from build123d import *
from build123d import SkipClean  # not in build123d's __all__

# Parameters (mm, degrees)
F1_DEPTH = 30.1625
F0_R     = 26.9169820067
F2_DEPTH = 38.1
F6_D     = 4.7625
F6_DEPTH = 114.301
F7_D     = 17.4625
F7_DEPTH = 19.0282397391


with BuildPart() as f1:
    # F0 (on Front) → F1 (new body, symmetric)
    with BuildSketch(Plane.XZ):
        with BuildLine():
            ThreePointArc((41.2750103626, 4.8735072878), (43.5200676937, 3.9435676542), (44.4499999995, 1.6985072878))
            Line((44.4499999995, 1.6985072878), (44.4499999995, 0))
            Line((44.4499999995, 0), (88.8999999995, 0))
            Line((88.8999999995, 0), (88.8999999995, 13.5279764081))
            ThreePointArc((88.8999999995, 13.5279764081), (88.0492603051, 16.7029781548), (85.7249965061, 19.0272397391))
            Line((85.7249965061, 19.0272397391), (47.6269838993, 19.0272397391))
            ThreePointArc((47.6269838993, 19.0272397391), (40.8967892902, 21.812053872), (38.1019943796, 28.5381099704))
            Line((38.1019943796, 28.5381099704), (38.0289897107, 77.7511383134))
            ThreePointArc((38.0289897107, 77.7511383134), (-2e-10, 39.7221486024), (-38.0289897112, 77.7511383134))
            Line((-38.0289897112, 77.7511383134), (-38.0289897112, 31.7225298162))
            ThreePointArc((-38.0289897112, 31.7225298162), (-40.8187976204, 24.9873377254), (-47.5539897112, 22.1975298162))
            Line((-47.5539897112, 22.1975298162), (-82.55, 22.1975298162))
            ThreePointArc((-82.55, 22.1975298162), (-87.0401280605, 20.3376578767), (-88.9, 15.8475298162))
            Line((-88.9, 15.8475298162), (-88.9, 0))
            Line((-88.9, 0), (-44.45, 0))
            Line((-44.45, 0), (-44.45, 1.6987767268))
            ThreePointArc((-44.45, 1.6987767268), (-43.5200603664, 3.943844421), (-41.274989637, 4.8737767268))
            Line((-41.274989637, 4.8737767268), (41.2750103626, 4.8735072878))
        make_face()
    extrude(amount=F1_DEPTH, both=True)

    # F0 (on Front) → F2 (join, symmetric)
    with BuildSketch(Plane.XZ):
        with BuildLine():
            ThreePointArc((-38.0289897112, 77.7511383134), (-2e-10, 39.7221486024), (38.0289897107, 77.7511383134))
            ThreePointArc((38.0289897107, 77.7511383134), (-2e-10, 115.7801280244), (-38.0289897112, 77.7511383134))
        make_face()
        with Locations((-2e-10, 77.7511383134)):
            Circle(F0_R, mode=Mode.SUBTRACT)
    with SkipClean():  # cleaning this boolean's faces spoils the solid; the shape is the same uncleaned
        extrude(amount=F2_DEPTH, both=True)

    # F6 (through all, one way)
    with BuildSketch(Plane.XY.offset(114.3)):
        with Locations((0, 0)):
            Circle(F6_D / 2)
    extrude(amount=-F6_DEPTH, mode=Mode.SUBTRACT)

    # F7 (through all, one way)
    with BuildSketch(Plane.XY.offset(19.0272397391)):
        with Locations((-66.6769838993, 0), (66.6769838993, 0)):
            Circle(F7_D / 2)
    extrude(amount=-F7_DEPTH, mode=Mode.SUBTRACT)


solid = f1.part
The listing builds one solid part. Answer for the finished solid, in the listing's coordinates (mm). A direction names the side the tool comes from. Give positions to 0.01 mm unless a question says otherwise; leave off trailing zeros. Loops run counter-clockwise (first coordinate to the right, second up) from the corner with the lowest first, then second, coordinate; pieces in that order, holes last. Notation, with made-up numbers: (74, 25.5) - (98, 25.5) arc R15 ccw to (98, 30.5) - close; hole circle Ø5 at (57, -27). An arc over 180 degrees is marked (long way). Write each question's results on one line, items separated by ' | '.
1. Find section A-A, the plane x = 0. Write down the section's boundary in (y, z).
Resolved:
outline: (-38.1, 39.72) - (-30.16, 39.72) - (-30.16, 4.87) - (-2.38, 4.87) - (-2.38, 50.83) - (-38.1, 50.83) - close; (-38.1, 104.67) - (-2.38, 104.67) - (-2.38, 114.3) - (2.38, 114.3) - (2.38, 104.67) - (38.1, 104.67) - (38.1, 115.78) - (-38.1, 115.78) - close; (2.38, 4.87) - (30.16, 4.87) - (30.16, 39.72) - (38.1, 39.72) - (38.1, 50.83) - (2.38, 50.83) - close
2. Find section D-D, the plane x = 23. Write down the section's boundary in (y, z).
Resolved:
outline: (-38.1, 47.47) - (-30.16, 47.47) - (-30.16, 4.87) - (30.16, 4.87) - (30.16, 47.47) - (38.1, 47.47) - (38.1, 63.77) - (-38.1, 63.77) - close; (-38.1, 91.73) - (38.1, 91.73) - (38.1, 108.04) - (-38.1, 108.04) - close
3. Flat-ended cylindrical pins translate along their axes: P1, Ø4, axis at x = 0, y = 0, coming from the -Z side; P2, Ø10, axis at y = 5.5, z = 91.5, coming from the -X side; P3, Ø1, axis at x = -27.5, y = 9.5, coming from the +Z side; P4, Ø14, axis at x = 66.68, y = 0, coming from the +Z side. Find the tip coordinate at first contact, or state that the pin passes through.
Resolved:
P1: stops at z = 114.3 | P2: stops at x = -37.01 | P3: stops at z = 104.53 | P4: passes through
4. For a pull along Y with two mould halves and no side action, classify faces 1 (the face through (0, 30.162, 22)), 2 (the face through (-1.89, -1.45, 28.23)), 3 (the face through (-67, 0, 19.027)), 4 (the face through (-26, -38.1, 70)) as +Y half, -Y half, draft (parallel to the pull), parting line (faces both ways), or undercut.
Resolved:
face 1: +Y half | face 2: undercut | face 3: undercut | face 4: -Y half
5. Consider probe 1 along Z at (x, y) = (0, -8); probe 2 along X at (y, z) = (1, 17); probe 3 along Z at (x, y) = (-53, 18). Determine where each line is inside the solid, lowest interval first. Write a range as from..to.
Resolved:
probe 1: z = 4.87..50.83, 104.67..115.78 | probe 2: x = -88.79..-75.35, -58..-2.16, 2.16..58, 75.35..87.87 | probe 3: z = 0..22.2
6. Find section C-C, the plane z = 58. Write down the section's boundary in (x, y), then the cut area to 3 significant figures.
Resolved:
outline: (-38.03, -30.16) - (-32.5, -30.16) - (-32.5, -38.1) - (-18.29, -38.1) - (-18.29, 38.1) - (-32.5, 38.1) - (-32.5, 30.16) - (-38.03, 30.16) - close; (18.29, -38.1) - (32.5, -38.1) - (32.5, -30.16) - (38.06, -30.16) - (38.06, 30.16) - (32.5, 30.16) - (32.5, 38.1) - (18.29, 38.1) - close | area: 2,830 mm^2
7. Which of the six approach directions +Z, -Z, +X, -X, +Y, -Y give full straight-line access (tool end or side, diameter ignored) to faces 5 (the face through (-88.9, 0, 8)), 6 (the face through (75, -7, 19.027)), 7 (the face through (-65, 0, 22.198)), 8 (the face through (-1.89, -1.45, 109.5)), 9 (the face through (-26, 38.1, 70))?
Resolved:
face 5: +Z, -Z, -X, +Y, -Y | face 6: +Z, +X, +Y, -Y | face 7: +Z, -X, +Y, -Y | face 8: -Z | face 9: +Z, -Z, +X, -X, +Y
